Part print with two shaded views. Sizes in mm from the minimum x, y, z corner. A direction names the side the tool comes from. Give positions to 0.01 mm unless a question says otherwise; leave off trailing zeros. Order: outer loops, then holes, each group sorted by start corner. A loop starts at its lowest first (then second) coordinate and runs counter-clockwise, first axis right, second up. Notation, with made-up numbers: (-19.75, 48) - (-4.75, 48) arc R21 ccw to (-4.75, 66) - close; hole circle Ø4 at (82, -13.5). An arc over 180 degrees is marked (long way). Return JSON: item names as keys, results as strings. Group by question number.
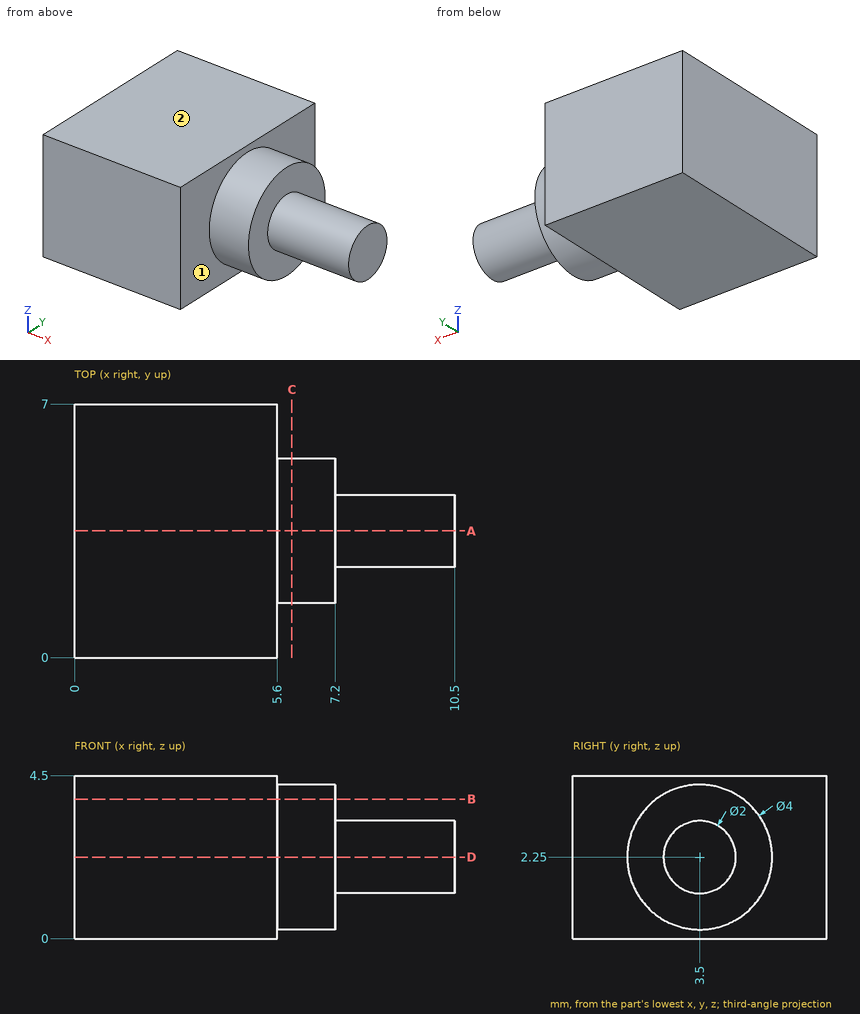
(1) Slice it at C-C (x = 6). Give the cut face in (y, z), and give its area (3 significant figures).
(2) 3-axis set-ups, long thin cutter, end or side, ignore diameter. For the marked faces 1 and 2: which of +Z, -Z, +X, -X, +Y, -Y reach the whole face in a straight line?
(3) Slice it at A-A (y = 3.5). Give the cut face in (x, z), and give its area (3 significant figures).
(4) Slice it at B-B (z = 3.85). Give the cut face in (x, y), and give its area (3 significant figures).
(5) Drill centre lines: L1, parallel to X at y = 4, z = 1.3; L2, parallel to X at y = 0.75, z = 0.6; L3, parallel to Z at x = 8, y = 3.5. Where is each one in solid material? Low to high.
(6) Slice it at D-D (z = 2.25). Give the cut face in (x, y).
Result set:
{
 "1": {"outline": "circle Ø4 at (3.5, 2.25)", "area": "12.6 mm²"},
 "2": {"face 1": "+X", "face 2": "+Z, +X, -X, +Y, -Y"},
 "3": {"outline": "(0, 0) - (5.6, 0) - (5.6, 0.25) - (7.2, 0.25) - (7.2, 1.25) - (10.5, 1.25) - (10.5, 3.25) - (7.2, 3.25) - (7.2, 4.25) - (5.6, 4.25) - (5.6, 4.5) - (0, 4.5) - close", "area": "38.2 mm²"},
 "4": {"outline": "(0, 0) - (5.6, 0) - (5.6, 2.3) - (7.2, 2.3) - (7.2, 4.7) - (5.6, 4.7) - (5.6, 7) - (0, 7) - close", "area": "43.0 mm²"},
 "5": {"L1": "x = 0 to 7.2", "L2": "x = 0 to 5.6", "L3": "z = 1.25 to 3.25"},
 "6": {"outline": "(0, 0) - (5.6, 0) - (5.6, 1.5) - (7.2, 1.5) - (7.2, 2.5) - (10.5, 2.5) - (10.5, 4.5) - (7.2, 4.5) - (7.2, 5.5) - (5.6, 5.5) - (5.6, 7) - (0, 7) - close"}
}
